```python
from build123d import *

# Parameters (mm, degrees)
BOSS_EXTRUDE1_DEPTH            = 7
SCREWHEADCLEARANCE_DEPTH       = 4
PCB_CUTOUT_DEPTH               = 30.03484975
SKETCH8_R                      = 1.25
SCREWTHREADS_DEPTH             = 16
SKETCH9_R                      = 3
CUT_EXTRUDE6_DEPTH             = 8.1
SKETCH10_W                     = 40
SKETCH10_H                     = 6.5
CUT_EXTRUDE7_DEPTH             = 30.034849842
FILLET1_R                      = 2
SKETCH11_R                     = 1.5
CLEARANCEHOLES_DEPTH           = 3
CLEARANCEHOLES_DRAFT           = -20
CLEARANCEHOLES_PROFILE_2_DEPTH = 3
CLEARANCEHOLES_PROFILE_2_DRAFT = -20
CLEARANCEHOLES_PROFILE_3_DEPTH = 3
CLEARANCEHOLES_PROFILE_3_DRAFT = -20


with BuildPart() as part:
    # Sketch1 → Boss-Extrude1 (new body)
    with BuildSketch(Plane.XY):
        with BuildLine():
            Line((0, 0), (18, 0))
            ThreePointArc((18, 0), (19.414213562, 0.585786438), (20, 2))
            Line((20, 2), (20, 11.945768163))
            ThreePointArc((20, 11.945768163), (19.769252649, 12.878369398), (19.130254936, 13.595775369))
            Line((19.130254936, 13.595775369), (10.510938386, 19.500007206))
            ThreePointArc((10.510938386, 19.500007206), (9.972285338, 19.760499203), (9.380683449, 19.85))
            Line((9.380683449, 19.85), (-9.380683449, 19.85))
            ThreePointArc((-9.380683449, 19.85), (-9.972285338, 19.760499203), (-10.510938386, 19.500007206))
            Line((-10.510938386, 19.500007206), (-19.130254936, 13.595775369))
            ThreePointArc((-19.130254936, 13.595775369), (-19.769252649, 12.878369398), (-20, 11.945768163))
            Line((-20, 11.945768163), (-20, 2))
            ThreePointArc((-20, 2), (-19.414213562, 0.585786438), (-18, 0))
            Line((-18, 0), (0, 0))
        make_face()
        with BuildLine():
            Line((-13.75, 9.075), (-13.75, 4.625))
            ThreePointArc((-13.75, 4.625), (-15.375, 3), (-17, 4.625))
            Line((-17, 4.625), (-17, 9.075))
            ThreePointArc((-17, 9.075), (-15.375, 10.7), (-13.75, 9.075))
        make_face(mode=Mode.SUBTRACT)
        with BuildLine():
            Line((17, 9.075), (17, 4.625))
            ThreePointArc((17, 4.625), (15.375, 3), (13.75, 4.625))
            Line((13.75, 4.625), (13.75, 9.075))
            ThreePointArc((13.75, 9.075), (15.375, 10.7), (17, 9.075))
        make_face(mode=Mode.SUBTRACT)
    extrude(amount=BOSS_EXTRUDE1_DEPTH)

    # Sketch2 → ScrewHeadClearance (cut)
    with BuildSketch(Plane.XY.offset(7)):
        with BuildLine():
            Line((-18.375, 4.625), (-18.375, 9.075))
            ThreePointArc((-18.375, 9.075), (-15.375, 12.075), (-12.375, 9.075))
            Line((-12.375, 9.075), (-12.375, 4.625))
            ThreePointArc((-12.375, 4.625), (-15.375, 1.625), (-18.375, 4.625))
        make_face()
        with BuildLine():
            Line((12.375, 4.625), (12.375, 9.075))
            ThreePointArc((12.375, 9.075), (15.375, 12.075), (18.375, 9.075))
            Line((18.375, 9.075), (18.375, 4.625))
            ThreePointArc((18.375, 4.625), (15.375, 1.625), (12.375, 4.625))
        make_face()
    extrude(amount=-SCREWHEADCLEARANCE_DEPTH, mode=Mode.SUBTRACT)

    # Sketch6 → PCB Cutout (cut, through all)
    with BuildSketch(Plane.XY.offset(7)):
        Polygon((-13.5, 13.35), (-6.5, 13.35), (-6.5, 19.85), (6.5, 19.85), (6.5, 13.35), (13.5, 13.35), (13.5, 11.75), (-13.5, 11.75), align=None)
    extrude(amount=-PCB_CUTOUT_DEPTH, mode=Mode.SUBTRACT)

    # Sketch8 → ScrewThreads (cut)
    with BuildSketch(Plane(origin=(0, 19.85, 0), x_dir=(1, 0, 0), z_dir=(0, 1, 0))):
        with Locations(Location((-10, -3.5, 0), (0, 0, 180))):
            Circle(SKETCH8_R)
        with Locations(Location((10, -3.5, 0), (0, 0, 180))):
            Circle(SKETCH8_R)
    extrude(amount=-SCREWTHREADS_DEPTH, mode=Mode.SUBTRACT)

    # Sketch9 → Cut-Extrude6 (cut)
    with BuildSketch(Plane(origin=(0, 19.85, 0), x_dir=(1, 0, 0), z_dir=(0, 1, 0))):
        with Locations(Location((10, -3.5, 0), (0, 0, 101.913740948))):
            Circle(SKETCH9_R)
        with Locations(Location((-10, -3.5, 0), (0, 0, 99.806006121))):
            Circle(SKETCH9_R)
    extrude(amount=-CUT_EXTRUDE6_DEPTH, mode=Mode.SUBTRACT)

    # Sketch10 → Cut-Extrude7 (cut, through all)
    with BuildSketch(Plane.XY.offset(7)):
        with Locations((0, 16.6)):
            Rectangle(SKETCH10_W, SKETCH10_H)
    extrude(amount=-CUT_EXTRUDE7_DEPTH, mode=Mode.SUBTRACT)

    # Fillet1
    # the kernel refuses this fillet: 2 mm, written as the material it takes off along each edge
    with BuildSketch(Plane(origin=(-19.424125327, 13.35, 12.203143064), x_dir=(-0.27669557885699486, -0.9609576247894558, 0), z_dir=(0, 0, -1))) as fillet1_piece_1:
        with BuildLine():
            CenterArc((1.527866068, -1.92191525), FILLET1_R, 73.936914891, 90)
            Line((-0.394049182, -1.368524092), (-0.586240707, -1.313184976))
            Line((-0.586240707, -1.313184976), (-0.192191525, 0.055339116))
            Line((-0.192191525, 0.055339116), (-0.095535811, 0.175706883))
            ThreePointArc((-0.095535811, 0.175706883), (1.564088383, 0.357037942), (2.136596341, 0.192191525))
            Line((2.136596341, 0.192191525), (2.081257226, 0))
        make_face()
    extrude(amount=17.406286128, mode=Mode.SUBTRACT)
    with BuildSketch(Plane(origin=(19.424125327, 13.35, 12.203143064), x_dir=(-1, 0, 0), z_dir=(0, 0, -1))) as fillet1_piece_2:
        with BuildLine():
            CenterArc((1.424125327, -2), FILLET1_R, 90, 90)
            Line((-0.575874673, -2), (-0.775874673, -2))
            ThreePointArc((-0.775874673, -2), (-0.775874673, -1.404231837), (-0.142412533, 0.140423184))
            Line((-0.142412533, 0.140423184), (0, 0.2))
            Line((0, 0.2), (1.424125327, 0.2))
            Line((1.424125327, 0.2), (1.424125327, 0))
        make_face()
    extrude(amount=17.406286128, mode=Mode.SUBTRACT)


with BuildPart() as clearanceholes_tool:
    # Sketch11 → ClearanceHoles (with draft: the straight prism first)
    with BuildSketch(Plane(origin=(0, 11.75, 0), x_dir=(1, 0, 0), z_dir=(0, 1, 0))):
        with Locations((0, -3.5)):
            Circle(SKETCH11_R)
    extrude(amount=-CLEARANCEHOLES_DEPTH)
    # ClearanceHoles: the draft: its side faces are tilted about the plane it starts from
    clearanceholes_sides = [clearanceholes_tool.faces().sort_by_distance(p)[0] for p in [
        (-1.5, 10.25, 3.5),
    ]]
    draft(clearanceholes_sides, Plane(origin=(0, 11.75, 0), x_dir=(1, 0, 0), z_dir=(0, 1, 0)), CLEARANCEHOLES_DRAFT)


with BuildPart() as part_1:
    add(part.part)

    # ClearanceHoles: cut by clearanceholes_tool
    add(clearanceholes_tool.part, mode=Mode.SUBTRACT)


with BuildPart() as clearanceholes_profile_2_tool:
    # Sketch11 → ClearanceHoles profile 2 (with draft: the straight prism first)
    with BuildSketch(Plane(origin=(0, 11.75, 0), x_dir=(1, 0, 0), z_dir=(0, 1, 0))):
        with Locations((5, -3.5)):
            Circle(SKETCH11_R)
    extrude(amount=-CLEARANCEHOLES_PROFILE_2_DEPTH)
    # ClearanceHoles profile 2: the draft: its side faces are tilted about the plane it starts from
    clearanceholes_profile_2_sides = [clearanceholes_profile_2_tool.faces().sort_by_distance(p)[0] for p in [
        (3.5, 10.25, 3.5),
    ]]
    draft(clearanceholes_profile_2_sides, Plane(origin=(0, 11.75, 0), x_dir=(1, 0, 0), z_dir=(0, 1, 0)), CLEARANCEHOLES_PROFILE_2_DRAFT)


with BuildPart() as part_2:
    add(part_1.part)

    # ClearanceHoles profile 2: cut by clearanceholes_profile_2_tool
    add(clearanceholes_profile_2_tool.part, mode=Mode.SUBTRACT)


with BuildPart() as clearanceholes_profile_3_tool:
    # Sketch11 → ClearanceHoles profile 3 (with draft: the straight prism first)
    with BuildSketch(Plane(origin=(0, 11.75, 0), x_dir=(1, 0, 0), z_dir=(0, 1, 0))):
        with Locations((-5, -3.5)):
            Circle(SKETCH11_R)
    extrude(amount=-CLEARANCEHOLES_PROFILE_3_DEPTH)
    # ClearanceHoles profile 3: the draft: its side faces are tilted about the plane it starts from
    clearanceholes_profile_3_sides = [clearanceholes_profile_3_tool.faces().sort_by_distance(p)[0] for p in [
        (-6.5, 10.25, 3.5),
    ]]
    draft(clearanceholes_profile_3_sides, Plane(origin=(0, 11.75, 0), x_dir=(1, 0, 0), z_dir=(0, 1, 0)), CLEARANCEHOLES_PROFILE_3_DRAFT)


with BuildPart() as part_3:
    add(part_2.part)

    # ClearanceHoles profile 3: cut by clearanceholes_profile_3_tool
    add(clearanceholes_profile_3_tool.part, mode=Mode.SUBTRACT)


solid = part_3.part
```
CAD build for the part. Positions are in the model's coordinates, mm. A direction names the side the tool comes from. Round coordinates to 2 decimals unless told otherwise and drop trailing zeros. Order: outer loops, then holes, each group sorted by start corner. A loop starts at its lowest first (then second) coordinate and runs counter-clockwise, first axis right, second up. Notation, with made-up numbers: (80.5, 32.25) - (116.5, 32.25) arc R26 ccw to (116.5, 46.25) - close; hole circle Ø10 at (-8.75, -24). An arc over 180 degrees is marked (long way). Answer as CSV lines item,"result". Start each with the question number.
1. Saw through at A-A, the plane y = 8. Write the cut outline in (x, z) (3 decimals).
2. Pull direction X, two halves, no side cores. Call faces 4 (the face through (-19.43, 12.75, 3.55)), 5 (the face through (13, 7, 3)), 6 (the face through (0, 0, 3)): +X half, -X half, draft (parallel to the pull), parting line (faces both ways), or undercut.
3. Saw through at C-C, the plane x = -10. Write the cut outline in (y, z).
4. Saw through at D-D, the plane x = -5. Write the cut outline in (y, z).
5. Drill centre lines: L1, parallel to X at y = 8.25, z = 6.5 (3 decimals); L2, parallel to X at y = 6.75, z = 2; L3, parallel to Z at x = -10, y = 9.25. Where is each one in solid material? Low to high. Write a range as [from, to].
6. Pin check, flat tips, straight feed: pin 1 (4 mm diameter, centred on x = -11, z = 1.5, fed in from +Y); pin 2 (1.8 mm diameter, centred on x = 16, y = 4.5, fed in from +Z); pin 3 (0.7 mm diameter, centred on x = 5, z = 3.5, fed in from +Y); pin 4 (6.5 mm diameter, centred on x = -14, y = 6, fed in from +Z). Stop position of each tip, or through.
7. Saw through at B-B, the plane z = 5.75. Write the cut outline in (x, y) (3 decimals).
8. Tool access for faces 1 (the face through (18.375, 7, 5)), 2 (the face through (-15.4, 10.7, 1.5)), 3 (the face through (10, 3.85, 4)): list every direction of +Z, -Z, +X, -X, +Y, -Y with a clear straight run to the whole face (end or side of a thin tool).
Model answer:
1,outline,"(-20, 0) - (-17, 0) - (-17, 3) - (-18.375, 3) - (-18.375, 7) - (-20, 7) - close; (-13.75, 0) - (13.75, 0) - (13.75, 3) - (12.375, 3) - (12.375, 7) - (-12.375, 7) - (-12.375, 3) - (-13.75, 3) - close; (17, 0) - (20, 0) - (20, 7) - (18.375, 7) - (18.375, 3) - (17, 3) - close; hole circle Ø2.5 at (-10, 3.5); hole circle Ø2.5 at (10, 3.5)"
2,face 4,"-X half"
2,face 5,"undercut"
2,face 6,"draft"
3,outline,"(0, 0) - (11.75, 0) - (11.75, 2.25) - (3.85, 2.25) - (3.85, 4.75) - (11.75, 4.75) - (11.75, 7) - (0, 7) - close"
4,outline,"(0, 0) - (11.75, 0) - (11.75, 2) - (8.75, 3.09) - (8.75, 3.91) - (11.75, 5) - (11.75, 7) - (0, 7) - close"
5,L1,"x = [-20, -18.375], [-12.375, 12.375], [18.375, 20]"
5,L2,"x = [-20, -17], [-13.75, 13.75], [17, 20]"
5,L3,"z = [0, 2.25], [4.75, 7]"
6,pin 1,"stops at y = 11.75"
6,pin 2,"passes through"
6,pin 3,"stops at y = 8.75"
6,pin 4,"stops at z = 7"
7,outline,"(-20, 2) arc R2 ccw to (-18, 0) - (18, 0) arc R2 ccw to (20, 2) - (20, 11.35) arc R2 ccw to (18, 13.35) - (13.5, 13.35) - (13.5, 11.75) - (-13.5, 11.75) - (-13.5, 13.35) - (-18, 13.35) arc R2 ccw to (-20, 11.35) - close; hole (-18.375, 4.625) arc R3 ccw to (-12.375, 4.625) - (-12.375, 9.075) arc R3 ccw to (-18.375, 9.075) - close; hole (12.375, 4.625) arc R3 ccw to (18.375, 4.625) - (18.375, 9.075) arc R3 ccw to (12.375, 9.075) - close"
8,face 1,"+Z"
8,face 2,"+Z, -Z"
8,face 3,"+Y"
